from build123d import *

# Parameters (mm, degrees)
DODANIE_WYCI_GNI_CIE1_DEPTH = 2
SZKIC2_W                    = 10.16
SZKIC2_H                    = 2.54
DODANIE_WYCI_GNI_CIE2_DEPTH = 10


with BuildPart() as part:
    # Szkic1 → Dodanie-wyciągnięcie1 (new body)
    with BuildSketch(Plane.XY):
        with BuildLine():
            Line((-8.932319644, 11.49408284), (8.067680356, 11.49408284))
            ThreePointArc((8.067680356, 11.49408284), (9.481893919, 10.908296403), (10.067680356, 9.49408284))
            Line((10.067680356, 9.49408284), (10.067680356, -0.50591716))
            ThreePointArc((10.067680356, -0.50591716), (9.481893919, -1.920130722), (8.067680356, -2.50591716))
            Line((8.067680356, -2.50591716), (-8.932319644, -2.50591716))
            ThreePointArc((-8.932319644, -2.50591716), (-10.346533206, -1.920130722), (-10.932319644, -0.50591716))
            Line((-10.932319644, -0.50591716), (-10.932319644, 9.49408284))
            ThreePointArc((-10.932319644, 9.49408284), (-10.346533206, 10.908296403), (-8.932319644, 11.49408284))
        make_face()
    extrude(amount=DODANIE_WYCI_GNI_CIE1_DEPTH)

    # Szkic2 → Dodanie-wyciągnięcie2 (add)
    with BuildSketch(Plane.XY.offset(2)):
        with Locations((-0.352319644, 8.72408284)):
            Rectangle(SZKIC2_W, SZKIC2_H)
    extrude(amount=DODANIE_WYCI_GNI_CIE2_DEPTH)


solid = part.part
Check sheet for the modelled part. Datum: model origin and axes. Units: mm. A direction names the side the tool comes from. Round coordinates to 2 decimals unless told otherwise and drop trailing zeros. Loops run counter-clockwise (first coordinate to the right, second up) from the corner with the lowest first, then second, coordinate; pieces in that order, holes last. Notation, with made-up numbers: M -15,-39.75 L 23,-39.75 A25 cw 23,-18.75 Z; hole C -29.75,-30 d1. An arc over 180 degrees is marked long. One line per item, written item: value.
(1) Access from +Z, -Z, +X, -X, +Y, -Y to the whole of each face (thin tool, end or side, straight path). Record for faces 1 (the face through (0, 9.994, 7)), 2 (the face through (4.728, 9, 7)), 3 (the face through (-5.432, 9, 7)).
Computed values:
face 1: +Z, +X, -X, +Y
face 2: +Z, +X, +Y, -Y
face 3: +Z, -X, +Y, -Y
(2) Sectioned sample at C-C, the plane z = 3. Record the cut outline in (x, y), then the cut area to 3 significant figures.
Computed values:
outline: M -5.43,7.45 L 4.73,7.45 L 4.73,9.99 L -5.43,9.99 Z
area: 25.8 mm^2
(3) Depth check by flat-ended pin: pin 1 Ø3 at (x, z) = (-1.5, 6) entering from -Y; pin 2 Ø1.3 at (y, z) = (9, 8.5) entering from +X; pin 3 Ø0.8 at (y, z) = (9, 6) entering from -X. Enter the tip coordinate at first touch or a pass-through.
Computed values:
pin 1: stops at y = 7.45
pin 2: stops at x = 4.73
pin 3: stops at x = -5.43
(4) Thickness scan on line 1 (Y direction, x = 1.5, z = 5); line 2 (Z direction, x = 5, y = -1); line 3 (X direction, y = 8.25, z = 7.5). Record the ranges inside material, lowest first.
Computed values:
line 1: y = 7.45 to 9.99
line 2: z = 0 to 2
line 3: x = -5.43 to 4.73
(5) Sectioned sample at A-A, the plane x = -0.75. Record the cut outline in (y, z), then the cut area to 3 significant figures.
Computed values:
outline: M -2.51,0 L 11.49,0 L 11.49,2 L 9.99,2 L 9.99,12 L 7.45,12 L 7.45,2 L -2.51,2 Z
area: 53.4 mm^2
(6) Sectioned sample at B-B, the plane y = 3.5. Record the cut outline in (x, z), then the cut area to 3 significant figures.
Computed values:
outline: M -10.93,0 L 10.07,0 L 10.07,2 L -10.93,2 Z
area: 42.0 mm^2
